The listing builds one solid part. Answer for the finished solid, in the listing's coordinates (mm). Coordinates: 2 decimals unless noted, no trailing zeros. Loops run counter-clockwise (first coordinate to the right, second up) from the corner with the lowest first, then second, coordinate; pieces in that order, holes last. Notation, with made-up numbers: (38, -20) - (49, -20) arc R22 ccw to (49, 9) - close; hole circle Ø1 at (-31, 69.25). An arc over 180 degrees is marked (long way). One line per question, with ' | ' between items.
from build123d import *

# Parameters (mm, degrees)
F0_W       = 0.508
F0_H       = 0.508
F1_DEPTH   = 4.5
F2_DEPTH   = 1.27
F3_DEPTH   = 2.54
F4_DEPTH   = 6.35
F2_FACE1_W = 0.508
F2_FACE1_H = 0.508
F6_ANGLE   = 90
F7_DEPTH   = 6.35
F3_FACE1_W = 0.508
F3_FACE1_H = 0.508
F9_ANGLE   = 90
F10_DEPTH  = 6.35


with BuildPart() as f1:
    # F0 (on Top) → F1 (new body)
    with BuildSketch(Plane.XY):
        with BuildLine():
            Line((0, -1.778), (1.4368409794, -1.778))
            ThreePointArc((1.4368409794, -1.778), (0, 2.286), (-1.4368409794, -1.778))
            Line((-1.4368409794, -1.778), (0, -1.778))
        make_face()
        with Locations((-1.27, -0.381)):
            Rectangle(F0_W, F0_H, mode=Mode.SUBTRACT)
        with Locations((0, -0.381)):
            Rectangle(F0_W, F0_H, mode=Mode.SUBTRACT)
        with Locations((1.27, -0.381)):
            Rectangle(F0_W, F0_H, mode=Mode.SUBTRACT)
        with Locations((-1.27, -0.381)):
            Rectangle(F0_W, F0_H)
        with Locations((0, -0.381)):
            Rectangle(F0_W, F0_H)
        with Locations((1.27, -0.381)):
            Rectangle(F0_W, F0_H)
    extrude(amount=F1_DEPTH)

    # F0 (on Top) → F2 (join)
    with BuildSketch(Plane.XY):
        with Locations((1.27, -0.381)):
            Rectangle(F0_W, F0_H)
    extrude(amount=-F2_DEPTH)

    # F0 (on Top) → F3 (join)
    with BuildSketch(Plane.XY):
        with Locations((0, -0.381)):
            Rectangle(F0_W, F0_H)
    extrude(amount=-F3_DEPTH)

    # F0 (on Top) → F4 (join)
    with BuildSketch(Plane.XY):
        with Locations((-1.27, -0.381)):
            Rectangle(F0_W, F0_H)
    extrude(amount=-F4_DEPTH)

    # F2_face1 (on face) → F6 (revolve)
    with BuildSketch(Plane(origin=(1.27, -0.381, -1.27), x_dir=(1, 0, 0), z_dir=(0, 0, -1))):
        Rectangle(F2_FACE1_W, F2_FACE1_H)
    revolve(axis=Axis((1.524, -1.0414, -1.27), (-1, 0, 0)), revolution_arc=F6_ANGLE)

    # F7 (add): a face of the model
    f7_faces = [f1.faces().sort_by_distance(p)[0] for p in [
        (1.27, -1.0414, -1.9304),
    ]]
    extrude(f7_faces, amount=F7_DEPTH)

    # F3_face1 (on face) → F9 (revolve)
    with BuildSketch(Plane(origin=(0, -0.381, -2.54), x_dir=(1, 0, 0), z_dir=(0, 0, -1))):
        Rectangle(F3_FACE1_W, F3_FACE1_H)
    revolve(axis=Axis((0.6604, -0.635, -2.54), (0, -1, 0)), revolution_arc=F9_ANGLE)

    # F10 (add): a face of the model
    f10_faces = [f1.faces().sort_by_distance(p)[0] for p in [
        (0.6604, -0.381, -3.2004),
    ]]
    extrude(f10_faces, amount=F10_DEPTH)


solid = f1.part
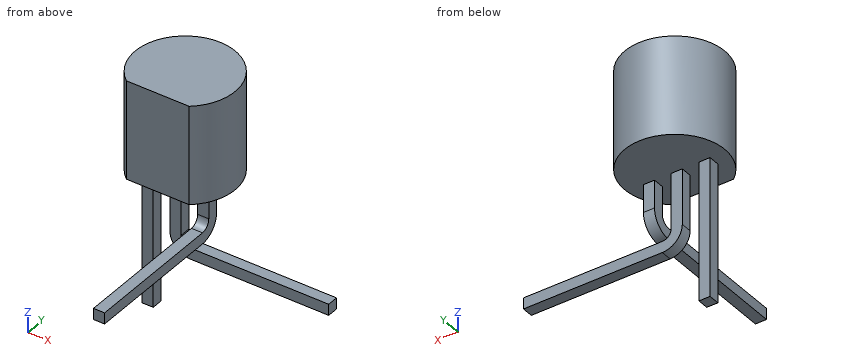
Item 1: Each of these flat-tipped pins is pushed along its axis until it touches: pin 1 Ø5 at (y, z) = (0, -3) entering from -X; pin 2 Ø0.6 at (x, z) = (1.5, -0.5) entering from +Y; pin 3 Ø0.6 at (x, z) = (-1.5, -3.5) entering from -Y (3 decimals); pin 4 Ø1 at (x, z) = (5.5, -2) entering from +Y. Where does it stop, or does it pass through?
Taken from the geometry:
pin 1: stops at x = -1.52 | pin 2: stops at y = -0.13 | pin 3: stops at y = -0.635 | pin 4: passes through
Item 2: Find section B-B, the plane z = -4.75. Write down the section's boundary in (x, y) (3 decimals), plus the area to 3 significant figures.
Taken from the geometry:
outline: (-1.524, -0.635) - (-1.016, -0.635) - (-1.016, -0.127) - (-1.524, -0.127) - close | area: 0.258 mm2
Item 3: Find the intervals of material crossed by line 1 (Z direction, x = 1.25, y = -5.25); line 2 (Z direction, x = -0.75, y = -1.5); line 3 (Y direction, x = 0.75, z = -3) (3 decimals), in increasing order. Write a range as [from, to].
Taken from the geometry:
line 1: z = [-2.18, -1.68] | line 2: z = [0, 4.5] | line 3: y = [-0.635, -0.127]
Item 4: Find section C-C, the plane y = -2. Write down the section's boundary in (x, z), plus the area to 3 significant figures.
Taken from the geometry:
outline: (1.02, -2.18) - (1.52, -2.18) - (1.52, -1.68) - (1.02, -1.68) - close | area: 0.258 mm2
Item 5: Find section D-D, the plane z = 0.5. Write down the section's boundary in (x, y).
Taken from the geometry:
outline: (-1.44, -1.78) - (1.44, -1.78) arc R2.29 ccw (long way) to start
Item 6: Find section A-A, the plane x = 0. Write down the section's boundary in (y, z) (3 decimals), plus the area to 3 significant figures.
Taken from the geometry:
outline: (-1.778, 0) - (-0.635, 0) - (-0.635, -3.172) - (-0.127, -3.172) - (-0.127, 0) - (2.286, 0) - (2.286, 4.5) - (-1.778, 4.5) - close | area: 19.9 mm2
